Geometry: final body of the model. Coordinates: model frame, mm. Face numbers are marked on the shaded views. A direction names the side the tool comes from. Give positions to 0.01 mm unless a question says otherwise; leave off trailing zeros. Write each loop counter-clockwise with the first axis right and the second up, starting at its lowest first coordinate (ties: lowest second). Pieces come first, ordered by that corner, then holes.
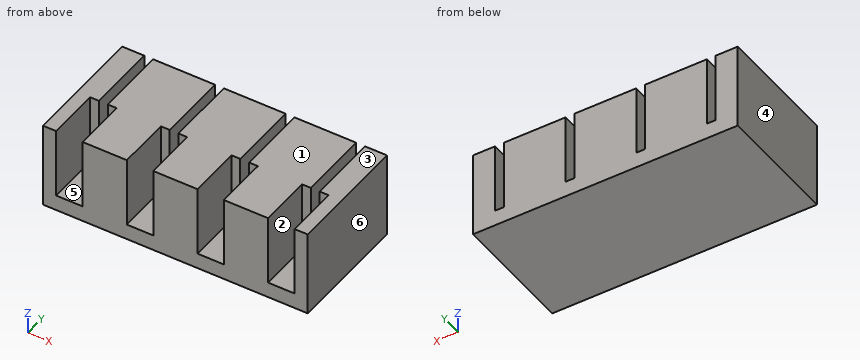
from build123d import *

# Parameters (mm, degrees)
F0_W     = 30
F0_H     = 14
F1_DEPTH = 9.8
F2_W     = 1
F2_H     = 14
F4_DEPTH = 8
F3_W     = 3
F3_H     = 6
F5_DEPTH = 8


with BuildPart() as f1:
    # F0 (on Top) → F1 (new body)
    with BuildSketch(Plane.XY):
        with Locations((-0.472123, 1.153064)):
            Rectangle(F0_W, F0_H)
    extrude(amount=F1_DEPTH)

    # F2 (on face) → F4 (cut)
    with BuildSketch(Plane.XY.offset(9.8)):
        with Locations((-12.472123, 1.153064)):
            Rectangle(F2_W, F2_H)
        with Locations((-4.472123, 1.153064)):
            Rectangle(F2_W, F2_H)
        with Locations((3.527877, 1.153064)):
            Rectangle(F2_W, F2_H)
        with Locations((11.527877, 1.153064)):
            Rectangle(F2_W, F2_H)
    extrude(amount=-F4_DEPTH, mode=Mode.SUBTRACT)

    # F3 (on face) → F5 (cut)
    with BuildSketch(Plane.XY.offset(9.8)):
        with Locations((-12.472123, -2.846936)):
            Rectangle(F3_W, F3_H)
        with Locations((-4.472123, -2.846936)):
            Rectangle(F3_W, F3_H)
        with Locations((3.527877, -2.846936)):
            Rectangle(F3_W, F3_H)
        with Locations((11.527877, -2.846936)):
            Rectangle(F3_W, F3_H)
    extrude(amount=-F5_DEPTH, mode=Mode.SUBTRACT)


solid = f1.part
Q1. Pin query (flat end, axial travel): P1, Ø0.5, axis at x = 12.5, z = 4.5, coming from the -Y side. Return the tip coordinate at first contact, or that it passes through.
Filled sheet:
P1: stops at y = 0.15
Q2. Section A-A on y = 6.5. Output: boundary loops of the cut face in (x, z).
Filled sheet:
outline: (-15.47, 0) - (14.53, 0) - (14.53, 9.8) - (12.03, 9.8) - (12.03, 1.8) - (11.03, 1.8) - (11.03, 9.8) - (4.03, 9.8) - (4.03, 1.8) - (3.03, 1.8) - (3.03, 9.8) - (-3.97, 9.8) - (-3.97, 1.8) - (-4.97, 1.8) - (-4.97, 9.8) - (-11.97, 9.8) - (-11.97, 1.8) - (-12.97, 1.8) - (-12.97, 9.8) - (-15.47, 9.8) - close
Q3. Section B-B on z = 8. Count the separate pieces of the cut face and the enclosed holes in it, plus the area to 3 significant figures.
Filled sheet:
separate pieces: 5
enclosed holes: 0
area: 316 mm2
Q4. Section D-D on y = -1. Output: boundary loops of the cut face in (x, z), plus the area to 3 significant figures.
Filled sheet:
outline: (-15.47, 0) - (14.53, 0) - (14.53, 9.8) - (13.03, 9.8) - (13.03, 1.8) - (10.03, 1.8) - (10.03, 9.8) - (5.03, 9.8) - (5.03, 1.8) - (2.03, 1.8) - (2.03, 9.8) - (-2.97, 9.8) - (-2.97, 1.8) - (-5.97, 1.8) - (-5.97, 9.8) - (-10.97, 9.8) - (-10.97, 1.8) - (-13.97, 1.8) - (-13.97, 9.8) - (-15.47, 9.8) - close
area: 198 mm2
Q5. Ray query, line 1 along X through (y, z) = (-4.25, 2.25); line 2 along X through (y, z) = (2.5, 9.25); line 3 along Z through (x, y) = (-13.5, -1.75). Return the intervals inside material, ascending.
Filled sheet:
line 1: x = -15.47 to -13.97, -10.97 to -5.97, -2.97 to 2.03, 5.03 to 10.03, 13.03 to 14.53
line 2: x = -15.47 to -12.97, -11.97 to -4.97, -3.97 to 3.03, 4.03 to 11.03, 12.03 to 14.53
line 3: z = 0 to 1.8
Q6. Section C-C on x = 11.75. Output: boundary loops of the cut face in (y, z), plus the area to 3 significant figures.
Filled sheet:
outline: (-5.85, 0) - (8.15, 0) - (8.15, 1.8) - (-5.85, 1.8) - close
area: 25.2 mm2
Q7. Access query for the marked faces 1 and 2. Directions: +Z, -Z, +X, -X, +Y, -Y. A direction counts if a zero-diameter tool reaches every point of the face in a straight line with its end or side. Return the directions, or none.
Filled sheet:
face 1: +Z, +X, -X, +Y, -Y
face 2: +Z, -Y
Q8. Pull-direction query (X, two-part tool) for the marked faces 3, 4, 5 and 6; classes: released by +X, released by -X, zero draft, split by the parting line, or undercut.
Filled sheet:
face 3: zero draft
face 4: released by -X
face 5: undercut
face 6: released by +X
